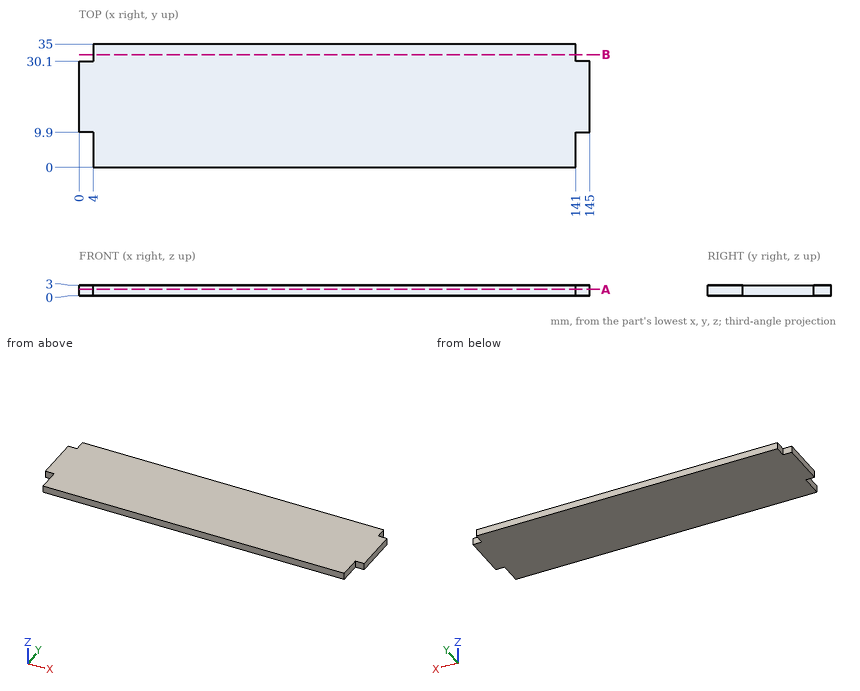
Could you check a few things on this drawing? It's one solid part, dimensions in mm from its lowest x, y, z. Coordinates: 2 decimals unless noted, no trailing zeros. Write each loop counter-clockwise with the first axis right and the second up, starting at its lowest first coordinate (ties: lowest second). Pieces come first, ordered by that corner, then holes.
1) If I drill on line 1 (X direction, y = 32, z = 1), over which ranges is the centre line in solid material (lowest first)?
Filled in:
line 1: x = 4 to 141
2) I'm going to push flat-ended pins straight in: pin 1 (0.9 mm diameter, centred on y = 32, z = 1, fed in from -X); pin 2 (1.5 mm diameter, centred on y = 33, z = 1.5, fed in from +X). Where does each tip first touch, or does it pass through?
Filled in:
pin 1: stops at x = 4
pin 2: stops at x = 141
3) If we section it at A-A (z = 1.85): List the corners of the cut face in (x, y) for me.
Filled in:
outline: (0, 9.9) - (4, 9.9) - (4, 0) - (141, 0) - (141, 9.9) - (145, 9.9) - (145, 30.1) - (141, 30.1) - (141, 35) - (4, 35) - (4, 30.1) - (0, 30.1) - close
4) If we section it at B-B (y = 32): List the corners of the cut face in (x, z) for me.
Filled in:
outline: (4, 0) - (141, 0) - (141, 3) - (4, 3) - close
